from build123d import *

# Parameters (mm, degrees)
SKETCH1_R                  = 53
BOSS_EXTRUDE1_DEPTH        = 50
F_10_0MM_DOWEL_HOLE1_D     = 10
F_10_0MM_DOWEL_HOLE1_DEPTH = 17.5
F_10_0MM_DOWEL_HOLE1_TIP   = 3.004303095
M4_TAPPED_HOLE1_REACH      = 130.627
M4_TAPPED_HOLE1_BORE_R     = 1.65
CIRPATTERN1_COUNT          = 3
CIRPATTERN1_ANGLE          = 180
SKETCH11_R                 = 30
CUT_EXTRUDE2_DEPTH         = 45
SKETCH12_W                 = 4.826
SKETCH12_H                 = 2.76515
SKETCH12_W_2               = 7.2136
SKETCH12_H_2               = 4.27264
SKETCH14_W                 = 2.667
SKETCH14_H                 = 4.572
SKETCH15_R                 = 4.5
CUT_EXTRUDE3_DEPTH         = 10
CIRPATTERN2_COUNT          = 4


with BuildPart() as part:
    # Sketch1 → Boss-Extrude1 (new body)
    with BuildSketch(Plane.XY):
        Circle(SKETCH1_R)
    extrude(amount=BOSS_EXTRUDE1_DEPTH)

    # Ø10.0mm Dowel Hole1
    with Locations(Plane.XY.offset(50)):
        with Locations((-37, 0), (37, 0), (0, -40)):
            Hole(F_10_0MM_DOWEL_HOLE1_D / 2, depth=F_10_0MM_DOWEL_HOLE1_DEPTH)
            with Locations((0, 0, -(F_10_0MM_DOWEL_HOLE1_DEPTH + F_10_0MM_DOWEL_HOLE1_TIP / 2))):  # 118° drill point
                Cone(0, F_10_0MM_DOWEL_HOLE1_D / 2, F_10_0MM_DOWEL_HOLE1_TIP, mode=Mode.SUBTRACT)

    # M4 Tapped Hole1 bore → M4 Tapped Hole1 (cut, up to next)
    with BuildSketch(Plane.ZY.offset(53), mode=Mode.PRIVATE) as m4_tapped_hole1_sk1:
        with Locations((44, 0)):
            Circle(M4_TAPPED_HOLE1_BORE_R)
    m4_tapped_hole1_tool1 = extrude(m4_tapped_hole1_sk1.sketch, amount=-M4_TAPPED_HOLE1_REACH, mode=Mode.PRIVATE) & part.part
    m4_tapped_hole1 = m4_tapped_hole1_tool1.solids().sort_by_distance((-53, 0, 44))[0]
    add(m4_tapped_hole1, mode=Mode.SUBTRACT)

    # CirPattern1: M4 Tapped Hole1 ×3 about axis
    cirpattern1_axis = Axis((0, 0, 50), (0, 0, 1))
    for i in range(1, CIRPATTERN1_COUNT):
        add(m4_tapped_hole1.rotate(cirpattern1_axis, i * CIRPATTERN1_ANGLE / (CIRPATTERN1_COUNT - 1)), mode=Mode.SUBTRACT)

    # Sketch11 → Cut-Extrude2 (cut)
    with BuildSketch(Plane.XY.offset(50)):
        Circle(SKETCH11_R)
    extrude(amount=-CUT_EXTRUDE2_DEPTH, mode=Mode.SUBTRACT)

    # Sketch12 → Cut-Revolve1 (revolve, cut)
    with BuildSketch(Plane(origin=(0, 0, 0), x_dir=(0, 0, -1), z_dir=(1, 0, 0)), mode=Mode.PRIVATE) as cut_revolve1_sk:
        with Locations((-12.413, 51.617425)):
            Rectangle(SKETCH12_W, SKETCH12_H)
        with Locations((-23.4328, 50.86368)):
            Rectangle(SKETCH12_W_2, SKETCH12_H_2)
    revolve(cut_revolve1_sk.sketch.rotate(Axis((0, 0, 0), (0, 0, 1)), 90), axis=Axis((0, 0, 0), (0, 0, 1)), mode=Mode.SUBTRACT)

    # Sketch14 → Cut-Revolve2 (revolve, cut)
    with BuildSketch(Plane(origin=(0, 0, 0), x_dir=(0, 0, -1), z_dir=(1, 0, 0)), mode=Mode.PRIVATE) as cut_revolve2_sk:
        with Locations((-1.3335, 24.8666)):
            Rectangle(SKETCH14_W, SKETCH14_H)
    revolve(cut_revolve2_sk.sketch.rotate(Axis((0, 0, 0), (0, 0, -1)), 270), axis=Axis((0, 0, 0), (0, 0, -1)), mode=Mode.SUBTRACT)

    # Sketch15 → Cut-Extrude3 (cut)
    with BuildSketch(Plane(origin=(0, 0, 0), x_dir=(-1, 0, 0), z_dir=(0, 0, -1))):
        with Locations((-10.606601718, 10.606601718)):
            Circle(SKETCH15_R)
        with Locations((0, -15)):
            Circle(SKETCH15_R)
        with Locations((10.606601718, 10.606601718)):
            Circle(SKETCH15_R)
    extrude(amount=-CUT_EXTRUDE3_DEPTH, mode=Mode.SUBTRACT)

    # Sketch17 → M5 Tapped Hole1 (revolve, cut)
    with BuildSketch(Plane(origin=(-28.284271247, 28.284271247, 0), x_dir=(0, 1, 0), z_dir=(1, 0, 0))):
        Polygon((0, 0), (0, 15.2618073), (2.1, 14), (2.1, 0), align=None)
    m5_tapped_hole1 = revolve(axis=Axis((-28.284271247, 28.284271247, -6.35), (0, 0, 1)), mode=Mode.SUBTRACT)

    # CirPattern2: M5 Tapped Hole1 ×4 about axis
    cirpattern2_axis = Axis((0, 0, 0), (0, 0, 1))
    for i in range(1, CIRPATTERN2_COUNT):
        add(m5_tapped_hole1.rotate(cirpattern2_axis, i * 360 / CIRPATTERN2_COUNT), mode=Mode.SUBTRACT)


solid = part.part
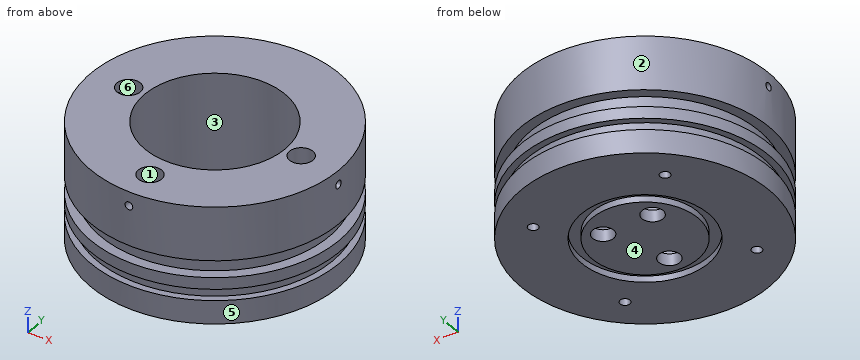
Here's how the part is built. I have some questions about the finished solid (model axes, mm). Face numbers are marked on the shaded views. A direction names the side the tool comes from. Give positions to 0.01 mm unless a question says otherwise; leave off trailing zeros. Loops run counter-clockwise (first coordinate to the right, second up) from the corner with the lowest first, then second, coordinate; pieces in that order, holes last. Notation, with made-up numbers: (27, -20) -> (36, -20) arc R16 cw to (36, -16) -> close; hole circle Ø10 at (-28.75, 11). An arc over 180 degrees is marked (long way). Answer as a JSON object with one key per item and string values. Group by question number.
Item 1: Imagine slicing it at A-A on z = 36.5. Write out the boundary of the cut face in (x, y).
Item 2: I need wall thicknesses on L1, parallel to Z at x = 40.5, y = 32.5; L2, parallel to Z at x = 43, y = 25; L3, parallel to Y at x = -4.5, z = 23. Which ranges of each line are inside material? Lowest first, please.
Item 3: Imagine slicing it at B-B on z = 44. Write out the boundary of the cut face in (x, y), then the cut area to 3 significant figures.
Item 4: Thinking about a two-plate mould opening in Y: for the marked faces 1, 2, 3 and 4, which applies, pulls with the +Y half, pulls with the -Y half, needs draft (parallel to the pull), parting line crosses it, or undercut?
Item 5: On a 3-axis mill with a long thin cutter (end or side, diameter ignored), from which of +Z, -Z, +X, -X, +Y, -Y can I reach the whole of each face in a straight line? I mean the marked faces 5 and 6. Say none if no direction works.
Item 6: Will these pins go through, and if not, where does the flat tip stop? pin 1 (8 mm diameter, centred on y = 15.5, z = 43.5, fed in from +X); pin 2 (10 mm diameter, centred on x = 40.5, z = 14.5, fed in from +Y); pin 3 (1.5 mm diameter, centred on x = -31, z = 32, fed in from -Y); pin 4 (10.5 mm diameter, centred on x = 10.61, y = 10.61, fed in from -Z).
Answer list:
{
 "1": {"outline": "circle Ø106 at (0, 0); hole circle Ø10 at (-37, 0); hole circle Ø60 at (0, 0); hole circle Ø10 at (0, -40); hole circle Ø10 at (37, 0)"},
 "2": {"L1": "z = 0 to 10, 14.83 to 19.83, 27.04 to 50", "L2": "z = 0 to 19.83, 27.04 to 50", "L3": "y = -48.52 to -29.66, 29.66 to 48.52"},
 "3": {"outline": "(-52.97, -1.65) arc R53 ccw to (-1.65, -52.97) -> (-1.65, -44.72) arc R5 cw (long way) to (1.65, -44.72) -> (1.65, -52.97) arc R53 ccw to (52.97, -1.65) -> (41.72, -1.65) arc R5 cw (long way) to (41.72, 1.65) -> (52.97, 1.65) arc R53 ccw to (-52.97, 1.65) -> (-41.72, 1.65) arc R5 cw (long way) to (-41.72, -1.65) -> close; hole circle Ø60 at (0, 0)", "area": "5,660 mm2"},
 "4": {"face 1": "undercut", "face 2": "parting line crosses it", "face 3": "undercut", "face 4": "needs draft"},
 "5": {"face 5": "+Z, -Z", "face 6": "+Z"},
 "6": {"pin 1": "stops at x = 51.74", "pin 2": "stops at y = 39.34", "pin 3": "stops at y = -43.52", "pin 4": "stops at z = 0"}
}
